Source: CAD feature listing. Evaluate the final solid. Frame: model axes, mm. A direction names the side the tool comes from. Coordinates: 2 decimals unless noted, no trailing zeros. Write each loop counter-clockwise with the first axis right and the second up, starting at its lowest first coordinate (ties: lowest second). Pieces come first, ordered by that corner, then holes. Notation, with made-up numbers: (72.25, 65.25) -> (95.25, 65.25) arc R9 cw to (95.25, 72.25) -> close; hole circle Ø3 at (9, -35). An arc over 180 degrees is marked (long way). Write item = value, one per line.
from build123d import *

# Parameters (mm, degrees)
SKETCH1_W           = 100
SKETCH1_H           = 116
BOSS_EXTRUDE1_DEPTH = 6
FILLET1_R           = 10
CUT_EXTRUDE1_DEPTH  = 6
SKETCH3_W           = 70
SKETCH3_H           = 54
BOSS_EXTRUDE2_DEPTH = 9
SKETCH5_R           = 8
BOSS_EXTRUDE3_DEPTH = 5


with BuildPart() as part:
    # Sketch1 → Boss-Extrude1 (new body)
    with BuildSketch(Plane(origin=(0, 0, 0), x_dir=(1, 0, 0), z_dir=(0, 1, 0))):
        Rectangle(SKETCH1_W, SKETCH1_H)
    extrude(amount=BOSS_EXTRUDE1_DEPTH)

    # Fillet1
    fillet1_edges = [part.edges().sort_by_distance(p)[0] for p in [
        (-50, 3, -58),
        (50, 3, -58),
        (50, 3, 58),
        (-50, 3, 58),
    ]]
    fillet(fillet1_edges, radius=FILLET1_R)

    # Sketch2 → Cut-Extrude1 (cut)
    with BuildSketch(Plane(origin=(0, 6, 0), x_dir=(1, 0, 0), z_dir=(0, 1, 0))):
        with BuildLine():
            Line((-36.189873482, 49.330370079), (-42.377057818, 41.198642095))
            ThreePointArc((-42.377057818, 41.198642095), (-41.330370079, 33.491214199), (-33.622942182, 34.537901938))
            Line((-33.622942182, 34.537901938), (-27.435757847, 42.669629921))
            ThreePointArc((-27.435757847, 42.669629921), (-28.482445586, 50.377057818), (-36.189873482, 49.330370079))
        make_face()
        with BuildLine():
            Line((36.189873482, 49.330370079), (42.377057818, 41.198642095))
            ThreePointArc((42.377057818, 41.198642095), (41.330370079, 33.491214199), (33.622942182, 34.537901938))
            Line((33.622942182, 34.537901938), (27.435757847, 42.669629921))
            ThreePointArc((27.435757847, 42.669629921), (28.482445586, 50.377057818), (36.189873482, 49.330370079))
        make_face()
        with BuildLine():
            Line((-36.189873482, -49.330370079), (-42.377057818, -41.198642095))
            ThreePointArc((-42.377057818, -41.198642095), (-41.330370079, -33.491214199), (-33.622942182, -34.537901938))
            Line((-33.622942182, -34.537901938), (-27.435757847, -42.669629921))
            ThreePointArc((-27.435757847, -42.669629921), (-28.482445586, -50.377057818), (-36.189873482, -49.330370079))
        make_face()
        with BuildLine():
            Line((36.189873482, -49.330370079), (42.377057818, -41.198642095))
            ThreePointArc((42.377057818, -41.198642095), (41.330370079, -33.491214199), (33.622942182, -34.537901938))
            Line((33.622942182, -34.537901938), (27.435757847, -42.669629921))
            ThreePointArc((27.435757847, -42.669629921), (28.482445586, -50.377057818), (36.189873482, -49.330370079))
        make_face()
    extrude(amount=-CUT_EXTRUDE1_DEPTH, mode=Mode.SUBTRACT)

    # Sketch3 → Boss-Extrude2 (add)
    with BuildSketch(Plane(origin=(0, 6, 0), x_dir=(1, 0, 0), z_dir=(0, 1, 0))):
        Rectangle(SKETCH3_W, SKETCH3_H)
    extrude(amount=BOSS_EXTRUDE2_DEPTH)

    # Sketch5 → Boss-Extrude3 (add)
    with BuildSketch(Plane.ZY.offset(35)):
        with BuildLine():
            Line((-27, 15), (27, 15))
            Line((27, 15), (27, 98.014328933))
            ThreePointArc((27, 98.014328933), (25.858192988, 103.754580418), (22.606601718, 108.62093065))
            Line((22.606601718, 108.62093065), (-17.36920564, 148.596738008))
            ThreePointArc((-17.36920564, 148.596738008), (-27.975807358, 152.990136291), (-38.582409076, 148.596738008))
            Line((-38.582409076, 148.596738008), (-55.552971824, 131.62617526))
            ThreePointArc((-55.552971824, 131.62617526), (-59.946370107, 121.019573542), (-55.552971824, 110.412971824))
            Line((-55.552971824, 110.412971824), (-31.393398282, 86.253398282))
            ThreePointArc((-31.393398282, 86.253398282), (-28.141807012, 81.38704805), (-27, 75.646796564))
            Line((-27, 75.646796564), (-27, 15))
        make_face()
        with Locations((-25.854487014, 118.898253199)):
            Circle(SKETCH5_R, mode=Mode.SUBTRACT)
    boss_extrude3 = extrude(amount=-BOSS_EXTRUDE3_DEPTH)

    # Mirror1: Boss-Extrude3 across plane
    add(boss_extrude3.mirror(Plane(origin=(0, 0, 0), x_dir=(0, 0, 1), z_dir=(1, 0, 0))))


solid = part.part
1) First-contact query: pin 1 Ø5 at (x, z) = (30.5, -48) entering from +Y; pin 2 Ø1.5 at (y, z) = (134.5, -39.5) entering from +X; pin 3 Ø8 at (x, y) = (32, 128.5) entering from -Z. Flat tips, straight axial feed; report the tip coordinate or a pass-through.
Answer block:
pin_1 = 141.68
pin_2 = 35
pin_3 = -59.54
2) Material intervals for probe 1 along X at (y, z) = (54, -7); probe 2 along Y at (x, z) = (-44, 20.5); probe 3 along Z at (x, y) = (33, 50), sorted ascending. Write a range as [from, to].
Answer block:
probe_1 = [-35, -30], [30, 35]
probe_2 = [0, 6]
probe_3 = [-27, 27]
3) Cut plane D-D, the plane z = 46. Output: boundary loops of the cut face in (x, y), and give its area (3 significant figures).
Answer block:
outline = (-50, 0) -> (-38.72, 0) -> (-38.72, 6) -> (-50, 6) -> close; (-26.31, 0) -> (26.31, 0) -> (26.31, 6) -> (-26.31, 6) -> close; (38.72, 0) -> (50, 0) -> (50, 6) -> (38.72, 6) -> close
area = 451 mm2
4) Cut plane B-B, the plane z = -46. Output: boundary loops of the cut face in (x, y), and give its area (3 significant figures).
Answer block:
outline = (-50, 0) -> (-38.72, 0) -> (-38.72, 6) -> (-50, 6) -> close; (-35, 100.86) -> (-30, 100.86) -> (-30, 141.18) -> (-35, 141.18) -> close; (-26.31, 0) -> (26.31, 0) -> (26.31, 6) -> (-26.31, 6) -> close; (30, 100.86) -> (35, 100.86) -> (35, 141.18) -> (30, 141.18) -> close; (38.72, 0) -> (50, 0) -> (50, 6) -> (38.72, 6) -> close
area = 854 mm2
5) Reachability of faces 4 (the flat face through (30.57, 3.04, 38.55)), 5 (the cylindrical face through (-28.387, 3.042, -50.303)), 6 (the cylindrical face through (-32.535, 81.463, -28.174)), 7 (the flat face through (-35, 81, -7)), 8 (the flat face through (0, 15, 0)) from +Z, -Z, +X, -X, +Y, -Y: full face, straight path, thin tool, end or side. Return the list, or none.
Answer block:
face_4 = +Y, -Y
face_5 = -Y
face_6 = -Z, +X, -X
face_7 = +Z, -Z, -X, +Y
face_8 = +Z, -Z, +Y
6) Cut plane C-C, the plane x = -38. Output: boundary loops of the cut face in (y, z).
Answer block:
outline = (0, -58) -> (6, -58) -> (6, -46.95) -> (0, -46.95) -> close; (0, -32.37) -> (6, -32.37) -> (6, 32.37) -> (0, 32.37) -> close; (0, 46.95) -> (6, 46.95) -> (6, 58) -> (0, 58) -> close
7) Cut plane A-A, the plane y = 33. Output: boundary loops of the cut face in (x, z), and give its area (3 significant figures).
Answer block:
outline = (-35, -27) -> (-30, -27) -> (-30, 27) -> (-35, 27) -> close; (30, -27) -> (35, -27) -> (35, 27) -> (30, 27) -> close
area = 540 mm2
8) Pull-direction query (X, two-part tool) for faces 1 (the flat face through (39.24, 3.04, 45.32)), 2 (the cylindrical face through (-32.53, 103.68, 25.89)), 3 (the flat face through (35, 81, -7)); classes: +X half, -X half, draft (parallel to the pull), parting line (faces both ways), or undercut.
Answer block:
face_1 = undercut
face_2 = draft
face_3 = +X half
